from build123d import *

# Parameters (mm, degrees)
SALIENTE_EXTRUIR1_DEPTH = 12
CROQUIS2_R              = 1.5
SALIENTE_EXTRUIR2_DEPTH = 6
CROQUIS3_R              = 1.5
CORTAR_EXTRUIR1_DEPTH   = 6


with BuildPart() as part:
    # Croquis1 → Saliente-Extruir1 (new body)
    with BuildSketch(Plane(origin=(0, 0, 0), x_dir=(1, 0, 0), z_dir=(0, 1, 0))):
        Polygon((0, 3.175426481), (-2.75, 1.58771324), (-2.75, -1.58771324), (0, -3.175426481), (2.75, -1.58771324), (2.75, 1.58771324), align=None)
    extrude(amount=SALIENTE_EXTRUIR1_DEPTH)

    # Croquis2 → Saliente-Extruir2 (add)
    with BuildSketch(Plane.XZ):
        Circle(CROQUIS2_R)
    extrude(amount=SALIENTE_EXTRUIR2_DEPTH)

    # Croquis3 → Cortar-Extruir1 (cut)
    with BuildSketch(Plane(origin=(0, 12, 0), x_dir=(1, 0, 0), z_dir=(0, 1, 0))):
        Circle(CROQUIS3_R)
    extrude(amount=-CORTAR_EXTRUIR1_DEPTH, mode=Mode.SUBTRACT)


solid = part.part
Verification items for the finished model (mm, model axes). A direction names the side the tool comes from. Coordinates: 2 decimals unless noted, no trailing zeros. Order: outer loops, then holes, each group sorted by start corner. A loop starts at its lowest first (then second) coordinate and runs counter-clockwise, first axis right, second up. Notation, with made-up numbers: M -19.75,-10.75 L 31.25,-10.75 A16 ccw 31.25,6.25 Z; hole C 29,-13 d1. An arc over 180 degrees is marked long. One line per item, written item: value. Start each with the question number.
Item 1: Sectioned sample at B-B on y = 2.25. Record the cut outline in (x, z), then the cut area to 3 significant figures.
Item 2: Mould release check, pull along Z, two halves, no side actions. Record for faces 1 (the cylindrical face through (-1.5, 9.04, -0.07)), 2 (the flat face through (-2.75, 6, 0)), 3 (the flat face through (1.36, 5.92, 2.39)): pulls with the +Z half, pulls with the -Z half, needs draft (parallel to the pull), parting line crosses it, or undercut.
Item 3: Sectioned sample at C-C on x = 0.2. Record the cut outline in (y, z), then the cut area to 3 significant figures.
Item 4: Depth check by flat-ended pin: P1, Ø1, axis at y = 6, z = 2, coming from the +X side; P2, Ø0.9, axis at x = 0.5, z = -0.5, coming from the +Y side; P3, Ø2, axis at x = -1, y = -2.5, coming from the +Z side. Enter the tip coordinate at first touch or a pass-through.
Item 5: Sectioned sample at A-A on z = 0. Record the cut outline in (x, y), then the cut area to 3 significant figures.
Item 6: Thickness scan on probe 1 along X at (y, z) = (10.6, 0); probe 2 along Y at (x, z) = (1.5, 1.5); probe 3 along Y at (x, z) = (-0.1, 0.5). Record the ranges inside material, lowest first.
Item 7: Sectioned sample at D-D on y = -0.25. Record the cut outline in (x, z), then the cut area to 3 significant figures.
Item 8: Access from +Z, -Z, +X, -X, +Y, -Y to the whole of each face (thin tool, end or side, straight path). Record for faces 4 (the flat face through (0, 6, 0)), 5 (the cylindrical face through (-1.5, -2.96, 0.07)), 6 (the flat face through (-1.36, 5.92, -2.39)).
Calculated:
1. outline: M -2.75,-1.59 L 0,-3.18 L 2.75,-1.59 L 2.75,1.59 L 0,3.18 L -2.75,1.59 Z
1. area: 26.2 mm^2
2. face 1: undercut
2. face 2: needs draft
2. face 3: pulls with the +Z half
3. outline: M -6,-1.49 L 0,-1.49 L 0,-3.06 L 12,-3.06 L 12,-1.49 L 6,-1.49 L 6,1.49 L 12,1.49 L 12,3.06 L 0,3.06 L 0,1.49 L -6,1.49 Z
3. area: 73.4 mm^2
4. P1: x = 2.75
4. P2: y = 6
4. P3: z = 1.5
5. outline: M -2.75,0 L -1.5,0 L -1.5,-6 L 1.5,-6 L 1.5,0 L 2.75,0 L 2.75,12 L 1.5,12 L 1.5,6 L -1.5,6 L -1.5,12 L -2.75,12 Z
5. area: 66.0 mm^2
6. probe 1: -2.75 to -1.5, 1.5 to 2.75
6. probe 2: 0 to 12
6. probe 3: -6 to 6
7. outline: C 0,0 d3
7. area: 7.07 mm^2
8. face 4: +Y
8. face 5: -Y
8. face 6: -Z, -X, +Y, -Y
